```python
from build123d import *

# Parameters (mm, degrees)
SKETCH1_R               = 100
SKETCH1_R_2             = 81.5
BOSS_EXTRUDE1_DEPTH     = 35
SKETCH3_R               = 27.5
CUT_EXTRUDE1_DEPTH      = 101
CUT_EXTRUDE1_DEPTH_BACK = 101
SKETCH4_R               = 5
CUT_EXTRUDE2_DEPTH      = 70
CIRPATTERN1_COUNT       = 8
CUT_EXTRUDE3_DEPTH      = 62


with BuildPart() as part:
    # Sketch1 → Boss-Extrude1 (new body, symmetric)
    with BuildSketch(Plane(origin=(0, 0, 0), x_dir=(1, 0, 0), z_dir=(0, 1, 0))):
        Circle(SKETCH1_R)
        Circle(SKETCH1_R_2, mode=Mode.SUBTRACT)
    extrude(amount=BOSS_EXTRUDE1_DEPTH, both=True)

    # Sketch3 → Cut-Extrude1 (cut, two sides)
    with BuildSketch(Plane.XY) as cut_extrude1_sk:
        with Locations((0, -2)):
            Circle(SKETCH3_R)
    extrude(amount=CUT_EXTRUDE1_DEPTH, mode=Mode.SUBTRACT)
    extrude(cut_extrude1_sk.sketch, amount=-CUT_EXTRUDE1_DEPTH_BACK, mode=Mode.SUBTRACT)

    # Sketch4 → Cut-Extrude2 (cut)
    with BuildSketch(Plane(origin=(0, 35, 0), x_dir=(1, 0, 0), z_dir=(0, 1, 0))):
        with Locations((-34.05882548, 82.225278394)):
            Circle(SKETCH4_R)
    cut_extrude2 = extrude(amount=-CUT_EXTRUDE2_DEPTH, mode=Mode.SUBTRACT)

    # CirPattern1: Cut-Extrude2 ×8 about axis
    cirpattern1_axis = Axis((0, 0, 0), (0, 1, 0))
    for i in range(1, CIRPATTERN1_COUNT):
        add(cut_extrude2.rotate(cirpattern1_axis, i * 360 / CIRPATTERN1_COUNT), mode=Mode.SUBTRACT)

    # Sketch5 → Cut-Extrude3 (cut)
    with BuildSketch(Plane.XZ.offset(35)):
        with BuildLine():
            Line((-72.5, -10), (72.5, -10))
            ThreePointArc((72.5, -10), (92.5, -30), (72.5, -50))
            Line((72.5, -50), (-72.5, -50))
            ThreePointArc((-72.5, -50), (-92.5, -30), (-72.5, -10))
        make_face()
    extrude(amount=-CUT_EXTRUDE3_DEPTH, mode=Mode.SUBTRACT)


solid = part.part
```
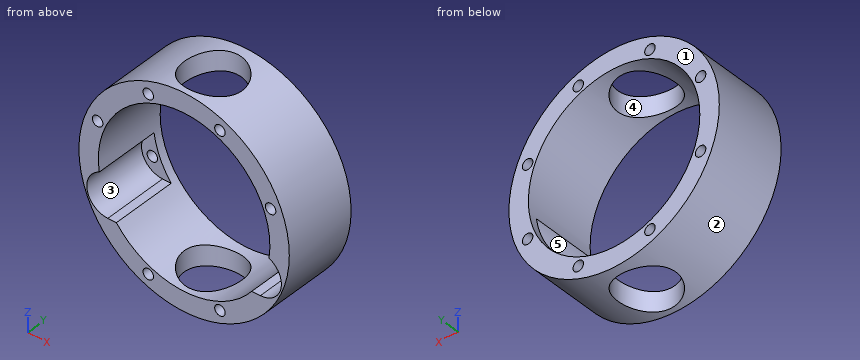
Can you work these out from the model? Positions are in its coordinate system, mm. Face numbers are marked on the shaded views. A direction names the side the tool comes from. Give positions to 0.01 mm unless a question says otherwise; leave off trailing zeros. Write each loop counter-clockwise with the first axis right and the second up, starting at its lowest first coordinate (ties: lowest second). Pieces come first, ordered by that corner, then holes. Notation, with made-up numbers: (48.25, 6) -> (65.25, 6) arc R20 cw to (65.25, 33) -> close; hole circle Ø6 at (25.5, 71). An arc over 180 degrees is marked (long way). Write item = value, one per line.
(1) Suppose I cut it at A-A on x = 0. Write out the boundary of the cut face in (y, z).
Worked out:
outline = (-35, -100) -> (-29.5, -100) -> (-29.5, -81.5) -> (-35, -81.5) -> close; (-35, 81.5) -> (-29.5, 81.5) -> (-29.5, 100) -> (-35, 100) -> close; (25.5, -100) -> (35, -100) -> (35, -81.5) -> (25.5, -81.5) -> close; (25.5, 81.5) -> (35, 81.5) -> (35, 100) -> (25.5, 100) -> close
(2) I'm going to push flat-ended pins straight in: P1, Ø14, axis at x = 84, z = -33.5, coming from the -Y side; P2, Ø5, axis at x = -58.5, y = -9.5, coming from the +Z side; P3, Ø10, axis at x = 24, y = -22, coming from the +Z side. Where does each tip first touch, or does it pass through?
Worked out:
P1 = 27
P2 = 82.85
P3 = 98.18
(3) Thinking about a two-plate mould opening in X: for the marked faces 1, 2 and 3, which applies, released by +X, released by -X, zero draft, split by the parting line, or undercut?
Worked out:
face_1 = zero draft
face_2 = split by the parting line
face_3 = undercut
(4) For the marked faces 4 and 5, which set-ups out of +Z, -Z, +X, -X, +Y, -Y let a thin tool reach every point of the face, with its end or its side?
Worked out:
face_4 = +Z, -Z
face_5 = -Y
(5) Suppose I cut it at B-B on y = -12. Write out the boundary of the cut face in (x, z).
Worked out:
outline = (-80.65, -11.74) arc R81.5 cw to (-25.62, 77.37) -> (-25.62, 96.66) arc R100 ccw to (-25.62, -96.66) -> (-25.62, -77.37) arc R81.5 cw to (-64.36, -50) -> (-72.5, -50) arc R20 cw to start; (25.62, -96.66) arc R100 ccw to (25.62, 96.66) -> (25.62, 77.37) arc R81.5 cw to (80.65, -11.74) arc R20 cw to (72.5, -50) -> (64.36, -50) arc R81.5 cw to (25.62, -77.37) -> close; hole circle Ø10 at (-82.23, 34.06); hole circle Ø10 at (-34.06, -82.23); hole circle Ø10 at (-34.06, 82.23); hole circle Ø10 at (34.06, -82.23); hole circle Ø10 at (34.06, 82.23); hole circle Ø10 at (82.23, 34.06)
(6) I need wall thicknesses on probe 1 along X at (y, z) = (-1.5, -1.5); probe 2 along Z at (x, y) = (34, -19); probe 3 along X at (y, z) = (-2, -85.5). Which ranges of each line are inside material? Lowest first, please. Write a range as from..to.
Worked out:
probe_1 = -99.99..-81.49, 81.49..99.99
probe_2 = -94.04..-87.22, -77.23..-74.07, 74.07..77.23, 87.22..94.04
probe_3 = -51.86..-37.84, -30.28..-27.5, 27.5..30.28, 37.84..51.86
(7) Suppose I cut it at D-D on y = 18.5. Write out the boundary of the cut face in (x, z).
Worked out:
outline = (-80.65, -11.74) arc R81.5 cw to (-18.33, 79.41) -> (-18.33, 98.31) arc R100 ccw to (-18.33, -98.31) -> (-18.33, -79.41) arc R81.5 cw to (-64.36, -50) -> (-72.5, -50) arc R20 cw to start; (18.33, -98.31) arc R100 ccw to (18.33, 98.31) -> (18.33, 79.41) arc R81.5 cw to (80.65, -11.74) arc R20 cw to (72.5, -50) -> (64.36, -50) arc R81.5 cw to (18.33, -79.41) -> close; hole circle Ø10 at (-82.23, 34.06); hole circle Ø10 at (-34.06, -82.23); hole circle Ø10 at (-34.06, 82.23); hole circle Ø10 at (34.06, -82.23); hole circle Ø10 at (34.06, 82.23); hole circle Ø10 at (82.23, 34.06)
(8) Suppose I cut it at C-C on z = 0. Write out the boundary of the cut face in (x, y).
Worked out:
outline = (-100, -35) -> (-81.5, -35) -> (-81.5, 35) -> (-100, 35) -> close; (81.5, -35) -> (100, -35) -> (100, 35) -> (81.5, 35) -> close
